Read the model definition and answer for the solid it produces. Units are mm, in the model's axes. Coordinates: 2 decimals unless noted, no trailing zeros. Loops run counter-clockwise (first coordinate to the right, second up) from the corner with the lowest first, then second, coordinate; pieces in that order, holes last.
from build123d import *

# Parameters (mm, degrees)
BOSS_EXTRUDE1_DEPTH = 175
FILLET1_R           = 10
SKETCH3_R           = 2
CUT_EXTRUDE1_DEPTH  = 340


with BuildPart() as part:
    # Sketch1 → Boss-Extrude1 (new, symmetric)
    with BuildSketch(Plane.XY):
        with BuildLine():
            Line((-56.291651246, 32.5), (-54.126587737, 31.25))
            ThreePointArc((-54.126587737, 31.25), (0, 62.5), (54.126587737, 31.25))
            Line((54.126587737, 31.25), (56.291651246, 32.5))
            ThreePointArc((56.291651246, 32.5), (0, 65), (-56.291651246, 32.5))
        make_face()
    extrude(amount=BOSS_EXTRUDE1_DEPTH, both=True)

    # Fillet1
    fillet1_edges = [part.edges().sort_by_distance(p)[0] for p in [
        (55.209119491, 31.875, 175),
        (55.209119491, 31.875, -175),
        (-55.209119491, 31.875, -175),
        (-55.209119491, 31.875, 175),
    ]]
    fillet(fillet1_edges, radius=FILLET1_R)

    # Sketch3 → Cut-Extrude1 (cut)
    with BuildSketch(Plane(origin=(0, 0, 0), x_dir=(1, 0, 0), z_dir=(0, 1, 0))):
        with Locations(Location((0, -170, 0), (0, 0, 90))):
            Circle(SKETCH3_R)
        with Locations(Location((0, 169, 0), (0, 0, 90))):
            Circle(SKETCH3_R)
    extrude(amount=CUT_EXTRUDE1_DEPTH, mode=Mode.SUBTRACT)


solid = part.part
Q1. A cutting plane is placed at A-A (y = 46.5). Give the vertices of the cut face in (x, z).
Findings below:
outline: (-45.42, -175) - (-41.76, -175) - (-41.76, 175) - (-45.42, 175) - close; (41.76, -175) - (45.42, -175) - (45.42, 175) - (41.76, 175) - close
Q2. A cutting plane is placed at B-B (z = 42.5). Give the vertices of the cut face in (x, y), then the cut area to 3 significant figures.
Findings below:
outline: (-56.29, 32.5) - (-54.13, 31.25) arc R62.5 cw to (54.13, 31.25) - (56.29, 32.5) arc R65 ccw to start
area: 334 mm2
Q3. Straight lines are drawn through the part: probe 1 along X at (y, z) = (34, -1); probe 2 along X at (y, z) = (38.5, -6.5); probe 3 along Y at (x, z) = (25, 119.5). For each, find the intervals that lie inside material, in ascending order.
Findings below:
probe 1: x = -55.4 to -52.44, 52.44 to 55.4
probe 2: x = -52.37 to -49.23, 49.23 to 52.37
probe 3: y = 57.28 to 60
Q4. Flat-ended cylindrical pins translate along their axes: pin 1 Ø8 at (x, z) = (-38, -127.5) entering from -Y; pin 2 Ø1.5 at (y, z) = (52, 14.5) entering from +X; pin 3 Ø5 at (x, z) = (-11, 52.5) entering from +Y; pin 4 Ø4.5 at (x, z) = (0, -169) entering from +Y. Find the tip coordinate at first contact, or state that the pin passes through.
Findings below:
pin 1: stops at y = 46.28
pin 2: stops at x = 39.98
pin 3: stops at y = 64.44
pin 4: stops at y = 65
Q5. Determine the mould class of faces 1 (the face through (-53.733, 34.315, 171.993)), 2 (the face through (-0.916, 62.493, 2.45)), 3 (the face through (53.773, 34.338, -171.993)), 4 (the face through (0, 63, -175)) for opening direction X: +X half, -X half, draft (parallel to the pull), parting line (faces both ways), or undercut.
Findings below:
face 1: -X half
face 2: undercut
face 3: +X half
face 4: draft
Q6. A cutting plane is placed at C-C (x = 8.5). Give the vertices of the cut face in (y, z), then the cut area to 3 significant figures.
Findings below:
outline: (61.92, -175) - (64.44, -175) - (64.44, 175) - (61.92, 175) - close
area: 883 mm2
